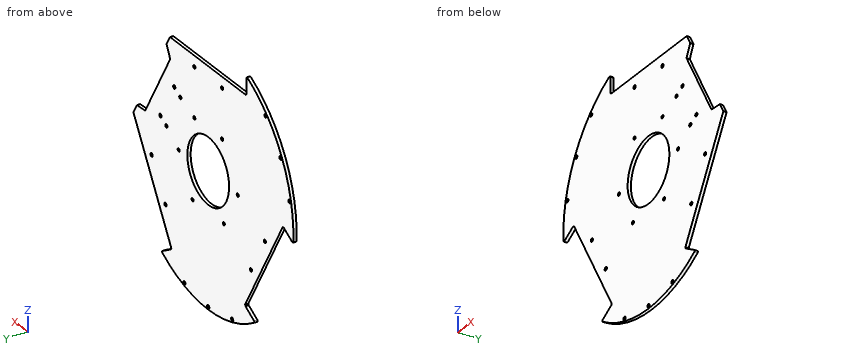
```python
from build123d import *

# Parameters (mm, degrees)
SKETCH_1_R          = 122.5
EXTRUDE_1_DEPTH     = 3
SKETCH_2_R          = 1.6
SKETCH_2_R_2        = 30
SKETCH_2_R_3        = 1.5
CUT_EXTRUDE_1_DEPTH = 174.267134795
CHAMFER_1_SIZE      = 1
FILLET_1_R          = 1


with BuildPart() as part:
    # ｽｹｯﾁ1 → ﾎﾞｽ - 押し出し1 (new body)
    with BuildSketch(Plane(origin=(0, 0, 0), x_dir=(1, 0, 0), z_dir=(0, 1, 0))):
        with Locations(Location((0, 0, 0), (0, 0, 270))):
            Circle(SKETCH_1_R)
    extrude(amount=EXTRUDE_1_DEPTH)

    # ｽｹｯﾁ2 → ｶｯﾄ - 押し出し1 (cut, through all)
    with BuildSketch(Plane(origin=(0, 3, 0), x_dir=(1, 0, 0), z_dir=(0, 1, 0))):
        with Locations(Location((20, -82.5, 0), (0, 0, 270))):
            Circle(SKETCH_2_R)
        with Locations(Location((-20, -82.5, 0), (0, 0, 270))):
            Circle(SKETCH_2_R)
        with Locations(Location((81.447095812, 23.929491924, 0), (0, 0, 270))):
            Circle(SKETCH_2_R)
        with Locations(Location((61.447095812, 58.570508076, 0), (0, 0, 270))):
            Circle(SKETCH_2_R)
        with Locations(Location((-61.447095812, 58.570508076, 0), (0, 0, 270))):
            Circle(SKETCH_2_R)
        with Locations(Location((-81.447095812, 23.929491924, 0), (0, 0, 270))):
            Circle(SKETCH_2_R)
        with Locations(Location((0, 0, 0), (0, 0, 270))):
            Circle(SKETCH_2_R_2)
        with Locations(Location((-42.475952642, 1.429491924, 0), (0, 0, 270))):
            Circle(SKETCH_2_R_3)
        with Locations(Location((-22.475952642, 36.070508076, 0), (0, 0, 270))):
            Circle(SKETCH_2_R_3)
        with Locations(Location((22.475952642, 36.070508076, 0), (0, 0, 270))):
            Circle(SKETCH_2_R_3)
        with Locations(Location((42.475952642, 1.429491924, 0), (0, 0, 270))):
            Circle(SKETCH_2_R_3)
        with Locations(Location((20, -37.5, 0), (0, 0, 270))):
            Circle(SKETCH_2_R_3)
        with Locations(Location((-20, -37.5, 0), (0, 0, 270))):
            Circle(SKETCH_2_R_3)
        with Locations(Location((-116.76259025, -27.685691575, 0), (0, 0, 270))):
            Circle(SKETCH_2_R)
        with Locations(Location((-103.923048454, -60, 0), (0, 0, 270))):
            Circle(SKETCH_2_R)
        with Locations(Location((-82.357807351, -87.276523581, 0), (0, 0, 270))):
            Circle(SKETCH_2_R)
        with Locations(Location((0, 120, 0), (0, 0, 270))):
            Circle(SKETCH_2_R)
        with Locations(Location((-34.4047829, 114.962215156, 0), (0, 0, 270))):
            Circle(SKETCH_2_R)
        with Locations(Location((34.4047829, 114.962215156, 0), (0, 0, 270))):
            Circle(SKETCH_2_R)
        with Locations(Location((48.787014427, -51.26120668, 0), (0, 0, 270))):
            Circle(SKETCH_2_R)
        with Locations(Location((68.787014427, -16.620190528, 0), (0, 0, 270))):
            Circle(SKETCH_2_R)
        with Locations(Location((40.126760389, -46.26120668, 0), (0, 0, 270))):
            Circle(SKETCH_2_R)
        with Locations(Location((60.126760389, -11.620190528, 0), (0, 0, 270))):
            Circle(SKETCH_2_R)
        Polygon((-55, -92.5), (55, -92.5), (60, -83.839745962), (54.656370753, -73.095183316), (90.630471022, -10.786213893), (102.60734985, -10.041651246), (107.60734985, -1.381397208), (52.60734985, 93.881397208), (104.568874077, 123.881397208), (159.568874077, 28.618602792), (55, -152.5), (-55, -152.5), align=None)
        Polygon((-104.568874077, 123.881397208), (-159.568874077, 28.618602792), (-107.60734985, -1.381397208), (-52.60734985, 93.881397208), align=None)
    extrude(amount=-CUT_EXTRUDE_1_DEPTH, mode=Mode.SUBTRACT)

    # 面取り1
    chamfer_1_edges = [part.edges().sort_by_distance(p)[0] for p in [
        (52.60734985, 1.5, -93.881397208),
        (-55, 1.5, 92.5),
        (-107.60734985, 1.5, 1.381397208),
        (-52.60734985, 1.5, -93.881397208),
    ]]
    chamfer(chamfer_1_edges, length=CHAMFER_1_SIZE)

    # ﾌｨﾚｯﾄ1
    fillet_1_edges = [part.edges().sort_by_distance(p)[0] for p in [
        (-55, 1.5, 109.458896395),
        (67.294184948, 1.5, -102.360845406),
        (-67.294184948, 1.5, -102.360845406),
        (-122.294184948, 1.5, -7.098050989),
    ]]
    fillet(fillet_1_edges, radius=FILLET_1_R)


solid = part.part
```
Geometry: final body of the model. Coordinates: model frame, mm. Coordinates: 2 decimals unless noted, no trailing zeros. Order: outer loops, then holes, each group sorted by start corner. A loop starts at its lowest first (then second) coordinate and runs counter-clockwise, first axis right, second up.
Item 1: Section query B-B (y = 1.2). State how many separate pieces and enclosed holes the cut face has, then the cut area to 3 significant figures.
Answer:
separate pieces: 1
enclosed holes: 23
area: 32,000 mm2
Item 2: Contact query for flat-ended pins moving along their axis: P1, Ø1.5, axis at y = 2, z = -91.5, coming from the -X side; P2, Ø1.5, axis at x = -60, y = 1.5, coming from the -Z side. Output: stop coordinate, or through.
Answer:
P1: stops at x = -54.42
P2: stops at z = -107.22
Item 3: Section query C-C (z = -69.5). Output: boundary loops of the cut face in (x, y).
Answer:
outline: (-66.68, 0) - (66.68, 0) - (66.68, 3) - (-66.68, 3) - close
Item 4: Section query A-A (x = -11). Output: boundary loops of the cut face in (y, z), then the cut area to 3 significant figures.
Answer:
outline: (0, -122.01) - (3, -122.01) - (3, -27.91) - (0, -27.91) - close; (0, 27.91) - (3, 27.91) - (3, 92.5) - (0, 92.5) - close
area: 476 mm2
Item 5: Material intervals for line 1 along X through (y, z) = (1.8, 27.5); line 2 along X through (y, z) = (2.4, 37.5); line 3 along Z through (x, y) = (56, 2.4), sorted ascending.
Answer:
line 1: x = -119.37 to -118.35, -115.17 to -11.99, 11.99 to 80.98
line 2: x = -116.62 to -21.5, -18.5 to 18.5, 21.5 to 75.21
line 3: z = -108.95 to -95.84, -88.01 to 70.77, 75.8 to 90.77
Item 6: Section query D-D (z = -42.5). Output: boundary loops of the cut face in (x, y).
Answer:
outline: (-82.27, 0) - (82.27, 0) - (82.27, 3) - (-82.27, 3) - close
